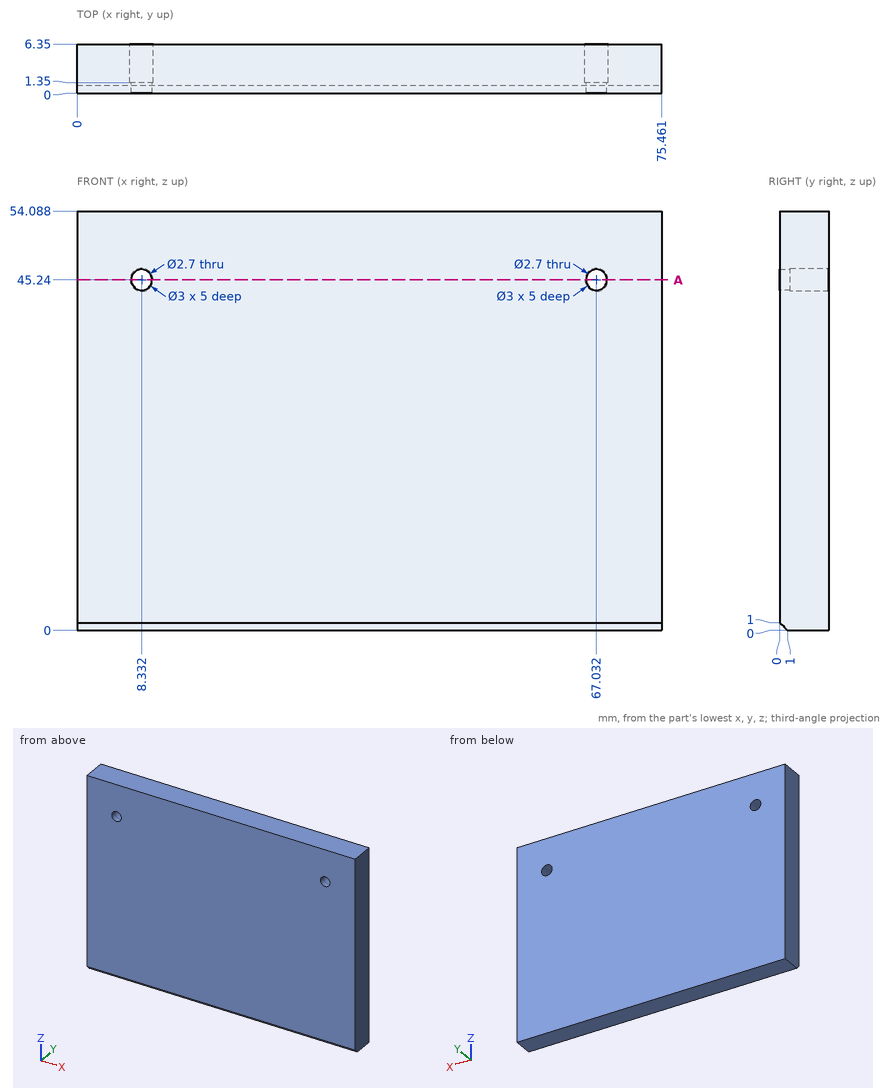
Study the drawing (mm; zero at the part's minimum x, y, z) and answer. Round coordinates to 2 decimals unless told otherwise and drop trailing zeros. Order: outer loops, then holes, each group sorted by start corner. A loop starts at its lowest first (then second) coordinate and runs counter-clockwise, first axis right, second up. Notation, with made-up numbers: M 8,-10 L 29,-10 A15 ccw 29,18 Z; hole C 27.25,-14 d7. An arc over 180 degrees is marked long. One line per item, written item: value.
Q1. Find section A-A on z = 45.24. Write down the section's boundary in (x, y), then the cut area to 3 significant figures.
Derived:
outline: M 0,0 L 6.98,0 L 6.98,1.35 L 6.83,1.35 L 6.83,6.35 L 0,6.35 Z; M 9.68,0 L 65.68,0 L 65.68,1.35 L 65.53,1.35 L 65.53,6.35 L 9.83,6.35 L 9.83,1.35 L 9.68,1.35 Z; M 68.38,0 L 75.46,0 L 75.46,6.35 L 68.53,6.35 L 68.53,1.35 L 68.38,1.35 Z
area: 442 mm²
Q2. A flat-ended cylindrical pin translates along its axis: pin 1 (1 mm diameter, centred on y = 1.5, z = 47, fed in from -X). Find the tip coordinate at first contact, or state that the pin passes through.
Derived:
pin 1: x = 0
Q3. Straight lines are drawn through the part: line 1 (X direction, y = 4.6, z = 45.24); line 2 (X direction, y = 1.15, z = 45.24). For each, find the intervals that lie inside material, in ascending order.
Derived:
line 1: 0 to 6.83, 9.83 to 65.53, 68.53 to 75.46
line 2: 0 to 6.98, 9.68 to 65.68, 68.38 to 75.46
